For this review, use the dimensioned drawing (mm, ordinates from the lowest corner) and the shaded views. A direction names the side the tool comes from. Round coordinates to 2 decimals unless told otherwise and drop trailing zeros. Write each loop counter-clockwise with the first axis right and the second up, starting at its lowest first coordinate (ties: lowest second). Pieces come first, ordered by that corner, then holes. Notation, with made-up numbers: (-20.5, -22.5) -> (-6.5, -22.5) arc R14 ccw to (-6.5, -15.5) -> close; hole circle Ø11 at (16, -1.5). An arc over 180 degrees is marked (long way). Answer as CSV lines item,"result". Start each with the question number.
Item 1: Take a section at B-B on z = 1.1. Give the boundary of the cut face in (x, y) (1 decimal).
Item 2: Wall thickness on probe 1 along Y at (x, z) = (3, 2.4); probe 2 along Z at (x, y) = (3, 1.25) (1 decimal); probe 3 along X at (y, z) = (3.75, 2.25) (1 decimal): over which ranges is each line inside the solid? List them lowest first. Write a range as from..to.
Item 3: Take a section at A-A on y = 6.75. Give the boundary of the cut face in (x, z) (1 decimal), then the cut area to 3 significant figures.
Item 4: Machinability: for the marked faces 1 and 2, which of the approach directions +Z, -Z, +X, -X, +Y, -Y give a long, thin tool a straight path to every point of the face, cutting with its end or side? Answer none if there is none.
Item 5: Take a section at C-C on x = 33. Give the boundary of the cut face in (y, z) (1 decimal).
Item 6: For pin 1 Ø1 at (y, z) = (3, 4) entering from -X (1 decimal); pin 2 Ø3 at (x, y) = (31, 3) entering from -Z; pin 3 Ø2 at (y, z) = (5.5, 3) entering from +X, all flat-tipped, find the tip position at first contact; note any pin that passes through.
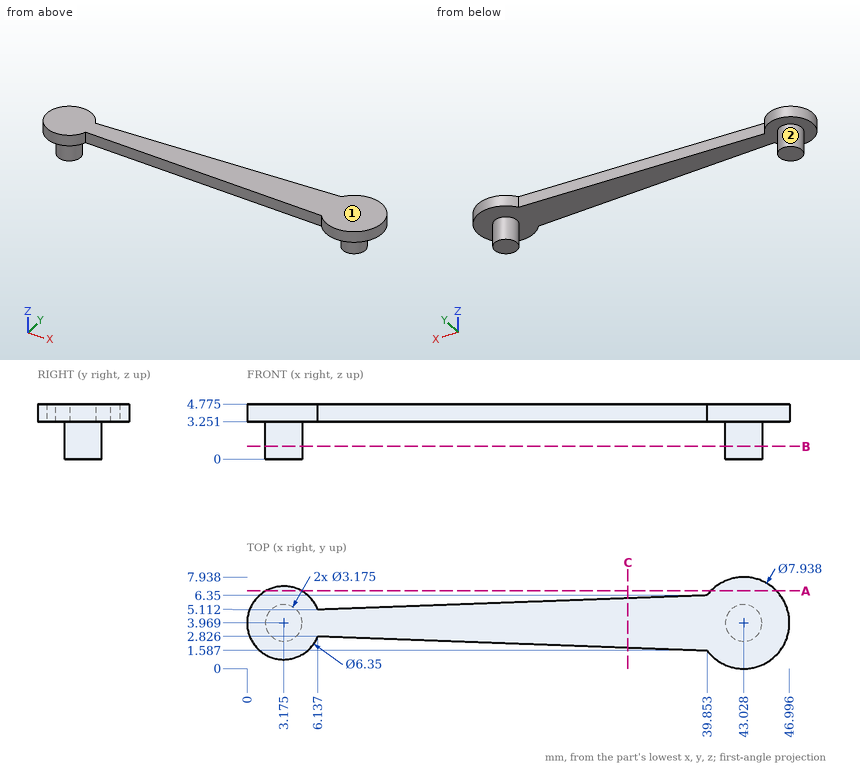
Output values:
1,outline,"circle Ø3.2 at (3.2, 4); circle Ø3.2 at (43, 4)"
2,probe 1,"y = 2.39..5.55"
2,probe 2,"z = 3.3..4.8"
2,probe 3,"x = 1.6..4.7, 41.5..44.6"
3,outline,"(1.6, 3.3) -> (4.7, 3.3) -> (4.7, 4.8) -> (1.6, 4.8) -> close; (40.2, 3.3) -> (45.9, 3.3) -> (45.9, 4.8) -> (40.2, 4.8) -> close"
3,area,"13.3 mm^2"
4,face 1,"+Z, +X, -X, +Y, -Y"
4,face 2,"-Z"
5,outline,"(1.8, 3.3) -> (6.1, 3.3) -> (6.1, 4.8) -> (1.8, 4.8) -> close"
6,pin 1,"stops at x = 0"
6,pin 2,"stops at z = 3.25"
6,pin 3,"stops at x = 46.96"
